The drawing under review shows one solid part. Ordinate dimensions are in mm from its lowest x, y, z. Coordinates: 2 decimals unless noted, no trailing zeros. Loops run counter-clockwise (first coordinate to the right, second up) from the corner with the lowest first, then second, coordinate; pieces in that order, holes last. Notation, with made-up numbers: (42.25, 7.25) - (55.25, 7.25) arc R19 ccw to (55.25, 40.25) - close; hole circle Ø6 at (71, -25). An arc over 180 degrees is marked (long way). Use one line per item in the form item = value. Start each with the question number.
1. Add section A-A on x = 45. Give the boundary of the cut face in (y, z).
2. Add section D-D on x = 13.5. Give the boundary of the cut face in (y, z).
3. To check wall thickness, follow probe 1 along X at (y, z) = (0.5, 12) (1 decimal); probe 2 along Z at (x, y) = (10, 4); probe 3 along Z at (x, y) = (19, 2.75). State the ranges of each line that lie inside material, in increasing order.
4. Draft analysis for pull direction X (two halves, no side actions). For the marked faces 1, 2, 3 and 4, state which applies: +X half, -X half, draft (parallel to the pull), parting line (faces both ways), or undercut.
5. Add section B-B on z = 27.5. Give the boundary of the cut face in (x, y).
6. Add section C-C on y = 1.5. Give the boundary of the cut face in (x, z) (1 decimal).
7. For pin 1 Ø3.5 at (x, z) = (10, 10.465) entering from -Y; pin 2 Ø3 at (x, y) = (11, 2.5) entering from +Z, all flat-tipped, find the tip position at first contact; note any pin that passes through.
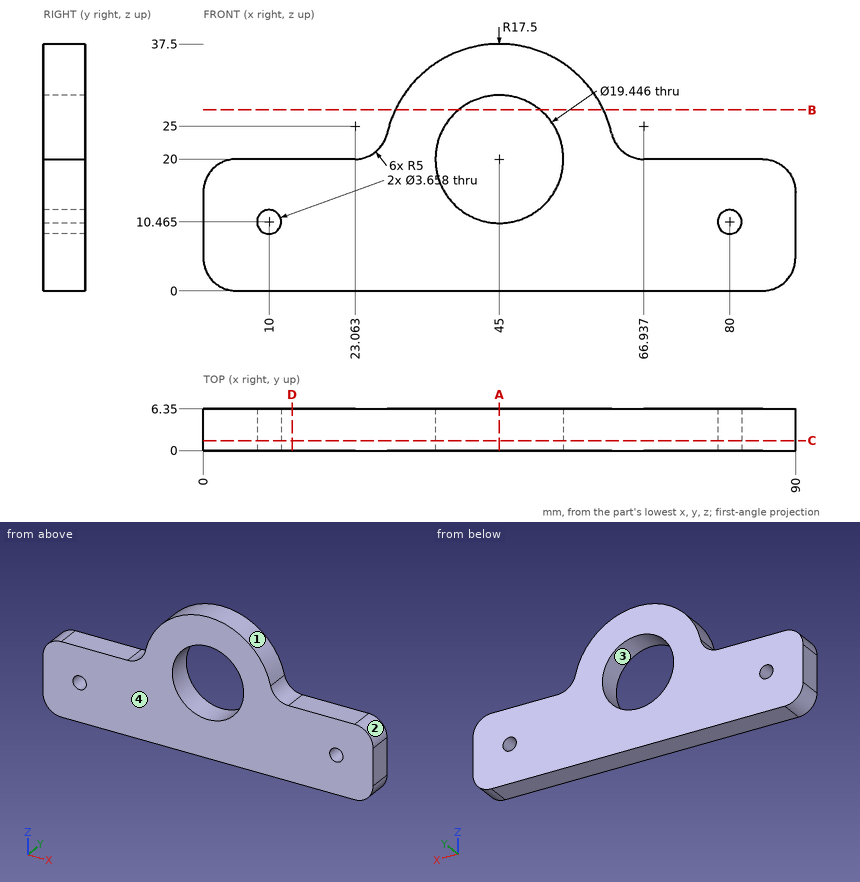
Conclusion:
q1.outline = (0, 0) - (6.35, 0) - (6.35, 10.28) - (0, 10.28) - close; (0, 29.72) - (6.35, 29.72) - (6.35, 37.5) - (0, 37.5) - close
q2.outline = (0, 0) - (6.35, 0) - (6.35, 20) - (0, 20) - close
q3.probe_1 = 0 to 9, 11 to 39.5, 50.5 to 79, 81 to 90
q3.probe_2 = 0 to 8.64, 12.29 to 20
q3.probe_3 = 0 to 20
q4.face_1 = parting line
q4.face_2 = +X half
q4.face_3 = undercut
q4.face_4 = draft
q5.outline = (29.19, 0) - (38.81, 0) - (38.81, 6.35) - (29.19, 6.35) - close; (51.19, 0) - (60.81, 0) - (60.81, 6.35) - (51.19, 6.35) - close
q6.outline = (0, 5) arc R5 ccw to (5, 0) - (85, 0) arc R5 ccw to (90, 5) - (90, 15) arc R5 ccw to (85, 20) - (66.9, 20) arc R5 cw to (62.1, 23.9) arc R17.5 ccw to (27.9, 23.9) arc R5 cw to (23.1, 20) - (5, 20) arc R5 ccw to (0, 15) - close; hole circle Ø3.7 at (10, 10.5); hole circle Ø19.4 at (45, 20); hole circle Ø3.7 at (80, 10.5)
q7.pin_1 = through
q7.pin_2 = 20
